Design review of the part built by this model. Coordinates are the model's own, in mm. A direction names the side the tool comes from. Give positions to 0.01 mm unless a question says otherwise; leave off trailing zeros. Loops run counter-clockwise (first coordinate to the right, second up) from the corner with the lowest first, then second, coordinate; pieces in that order, holes last. Notation, with made-up numbers: (85.5, 33.25) -> (138.5, 33.25) arc R22 cw to (138.5, 57.25) -> close; hole circle Ø10 at (15, -2). An arc over 180 degrees is marked (long way). Answer in a Markdown table with one row per item. Add a question column.
(1) Consider section C-C on y = -125.5. Write out the cut boundary in (x, z), then the cut area to 3 significant figures.
(2) Consider section A-A on y = 0. Write out the cut boundary in (x, z) (1 decimal).
(3) For line 1 (Y direction, x = 12, z = 5); line 2 (Y direction, x = 12.7, z = 5); line 3 (Z direction, x = 44, y = -56), list the stretches that pass through material, from the lowest coordinate up.
(4) Consider section D-D on y = 131. Write out the cut boundary in (x, z), then the cut area to 3 significant figures.
(5) Draft analysis for pull direction Z (two halves, no side actions). For faces 1 (the flat face through (147, 101, 12.7)), 2 (the flat face through (53, 32, 12.7)), 3 (the flat face through (106, 65, 101.6)), 4 (the flat face through (0, -57, 4)), state which applies: +Z half, -Z half, draft (parallel to the pull), parting line (faces both ways), or undercut.
(6) Consider section B-B on x = 12.7. Write out the cut boundary in (y, z).
(7) For faces 5 (the cylindrical face through (50.788, 1.117, 3.913)), 6 (the flat face through (50.654, 32.439, 56.528)), 7 (the flat face through (107, -32, 12.7)), 8 (the flat face through (140.32, 109.59, 56.53)), 9 (the cylindrical face through (12.01, 52.62, 3.91)), list the 3-axis set-ups (+Z, -Z, +X, -X, +Y, -Y) from which the entire face can be reached by the end or side of a thin tool; tool diameter is ignored.
(8) For pin 1 (8 mm diameter, centred on y = 31.5, z = 43, fed in from +X); pin 2 (2 mm diameter, centred on x = 81, z = 66.5, fed in from +Y); pin 3 (5 mm diameter, centred on x = 123.5, z = 18, fed in from -Y); pin 4 (5.5 mm diameter, centred on x = 57.15, y = 0, fed in from -Z), all flat-tipped, find the tip position at first contact; note any pin that passes through.
from build123d import *

# Parameters (mm, degrees)
F0_R     = 3.175
F1_DEPTH = 7.9375
F3_DEPTH = 12.7
F6_DEPTH = 88.9


with BuildPart() as f1:
    # F0 (on Top) → F1 (new body)
    with BuildSketch(Plane.XY):
        with BuildLine():
            ThreePointArc((0, 50.8), (50.8, 0), (0, -50.8))
            Line((0, -50.8), (0, -63.5))
            ThreePointArc((0, -63.5), (63.5, 0), (0, 63.5))
            Line((0, 63.5), (0, 50.8))
        make_face()
        with Locations((12.7, -55.7210238599)):
            Circle(F0_R, mode=Mode.SUBTRACT)
        with Locations((12.7, 55.7210238599)):
            Circle(F0_R, mode=Mode.SUBTRACT)
        with Locations((57.15, 0)):
            Circle(F0_R, mode=Mode.SUBTRACT)
    extrude(amount=F1_DEPTH)

    # F2 (on Top) → F3 (join)
    with BuildSketch(Plane.XY):
        with BuildLine():
            ThreePointArc((0, 63.5), (63.5, 0), (0, -63.5))
            Line((0, -63.5), (70.8477284562, -163.0749501689))
            ThreePointArc((70.8477284562, -163.0749501689), (177.8, 0), (70.8477284562, 163.0749501689))
            Line((70.8477284562, 163.0749501689), (0, 63.5))
        make_face()
    extrude(amount=F3_DEPTH)

    # F5 (on offset) → F6 (join)
    with BuildSketch(Plane.XY.offset(12.7)):
        with BuildLine():
            add(Edge.make_bspline(
                [(46.18588835, 41.1815866828), (59.2543137599, 45.7684123204), (86.0798549494, 55.1837838141), (130.6032472575, 83.2102673221), (130.0058690925, 109.2241975175), (129.7313123941, 121.1802735925)],
                knots=[0, 0, 0, 0, 0.3392119344, 0.6962999315, 1, 1, 1, 1], degree=3))
            Line((46.18588835, 41.1815866828), (55.2497804165, 23.447887972))
            add(Edge.make_bspline(
                [(55.2497804165, 23.447887972), (66.8035585634, 26.6415392462), (92.7958853953, 33.8262390606), (144.2666782475, 72.3809452741), (148.8411054612, 91.0665666373), (150.6176739931, 98.3234941959)],
                knots=[0, 0, 0, 0, 0.3286016832, 0.7392492948, 1, 1, 1, 1], degree=3))
            Line((150.6176739931, 98.3234941959), (129.7313123941, 121.1802735925))
        make_face()
    extrude(amount=F6_DEPTH)


solid = f1.part
Values follow:
| question | item | result |
|---|---|---|
| 1 | outline | (44.11, 0) -> (125.95, 0) -> (125.95, 12.7) -> (44.11, 12.7) -> close |
| 1 | area | 1,040 mm2 |
| 2 | outline | (50.8, 0) -> (54, 0) -> (54, 7.9) -> (50.8, 7.9) -> close; (60.3, 0) -> (177.8, 0) -> (177.8, 12.7) -> (63.5, 12.7) -> (63.5, 7.9) -> (60.3, 7.9) -> close |
| 3 | line 1 | -80.37 to -58.82, -52.62 to -49.36, 49.36 to 52.62, 58.82 to 80.37 |
| 3 | line 2 | -81.35 to -58.9, -52.55 to -49.19, 49.19 to 52.55, 58.9 to 81.35 |
| 3 | line 3 | 0 to 12.7 |
| 4 | outline | (48.03, 0) -> (120.22, 0) -> (120.22, 12.7) -> (48.03, 12.7) -> close |
| 4 | area | 917 mm2 |
| 5 | face 1 | -Z half |
| 5 | face 2 | undercut |
| 5 | face 3 | +Z half |
| 5 | face 4 | draft |
| 6 | outline | (-81.35, 0) -> (-58.9, 0) -> (-58.9, 7.94) -> (-62.22, 7.94) -> (-62.22, 12.7) -> (-81.35, 12.7) -> close; (-52.55, 0) -> (-49.19, 0) -> (-49.19, 7.94) -> (-52.55, 7.94) -> close; (49.19, 0) -> (52.55, 0) -> (52.55, 7.94) -> (49.19, 7.94) -> close; (58.9, 0) -> (81.35, 0) -> (81.35, 12.7) -> (62.22, 12.7) -> (62.22, 7.94) -> (58.9, 7.94) -> close |
| 7 | face 5 | +Z, -Z, -X |
| 7 | face 6 | +Z, -X, -Y |
| 7 | face 7 | +Z, +X, -Y |
| 7 | face 8 | +Z, +X, +Y |
| 7 | face 9 | +Z, -Z |
| 8 | pin 1 | x = 88.91 |
| 8 | pin 2 | y = 55.22 |
| 8 | pin 3 | y = 56.2 |
| 8 | pin 4 | through |
